from build123d import *
from OCP.BRepFilletAPI import BRepFilletAPI_MakeChamfer

# Parameters (mm, degrees)
BOSS_EXTRUDE1_DEPTH = 4.7625
CHAMFER1_SIZE       = 1.524
CHAMFER1_SIZE2      = 3.81
FILLET1_R           = 5.08


with BuildPart() as part:
    # Sketch1 → Boss-Extrude1 (new body)
    with BuildSketch(Plane.XY):
        with BuildLine():
            Line((-16.586093498, 9.370378993), (-35.326851484, -23.801808003))
            Line((-35.326851484, -23.801808003), (-2.154664488, -42.542565989))
            Line((-2.154664488, -42.542565989), (16.586093498, -9.370378993))
            ThreePointArc((16.586093498, -9.370378993), (9.370378993, 16.586093498), (-16.586093498, 9.370378993))
        make_face()
    extrude(amount=BOSS_EXTRUDE1_DEPTH)

    # Chamfer1: one chamfer whose edges measure the first distance from different faces: ONE call of the kernel's chamfer builder (chamfer() names one face for all edges)
    chamfer1_edges_1 = [part.edges().sort_by_distance(p)[0] for p in [
        (7.215714505, -25.956472491, 4.7625),
    ]]
    chamfer1_side_1 = [part.faces().sort_by_distance(p)[0] for p in [
        (7.215714505, -25.956472491, 2.38125),
    ]]
    chamfer1_edges_2 = [part.edges().sort_by_distance(p)[0] for p in [
        (9.370378993, 16.586093498, 4.7625),
    ]]
    chamfer1_side_2 = [part.faces().sort_by_distance(p)[0] for p in [
        (9.370378993, 16.586093498, 2.38125),
    ]]
    chamfer1_edges_3 = [part.edges().sort_by_distance(p)[0] for p in [
        (-25.956472491, -7.215714505, 4.7625),
    ]]
    chamfer1_side_3 = [part.faces().sort_by_distance(p)[0] for p in [
        (-25.956472491, -7.215714505, 2.38125),
    ]]
    chamfer1 = BRepFilletAPI_MakeChamfer(part.part.solid().wrapped)
    for e in chamfer1_edges_1:
        chamfer1.Add(CHAMFER1_SIZE, CHAMFER1_SIZE2, e.wrapped, chamfer1_side_1[0].wrapped)  # the first distance lies on this face
    for e in chamfer1_edges_2:
        chamfer1.Add(CHAMFER1_SIZE, CHAMFER1_SIZE2, e.wrapped, chamfer1_side_2[0].wrapped)  # the first distance lies on this face
    for e in chamfer1_edges_3:
        chamfer1.Add(CHAMFER1_SIZE, CHAMFER1_SIZE2, e.wrapped, chamfer1_side_3[0].wrapped)  # the first distance lies on this face
    add(Compound.cast(chamfer1.Shape()), mode=Mode.REPLACE)

    # Fillet1
    fillet1_edges = [part.edges().sort_by_distance(p)[0] for p in [
        (-35.326851484, -23.801808003, 1.61925),
        (-2.154664488, -42.542565989, 1.61925),
    ]]
    fillet(fillet1_edges, radius=FILLET1_R)


solid = part.part
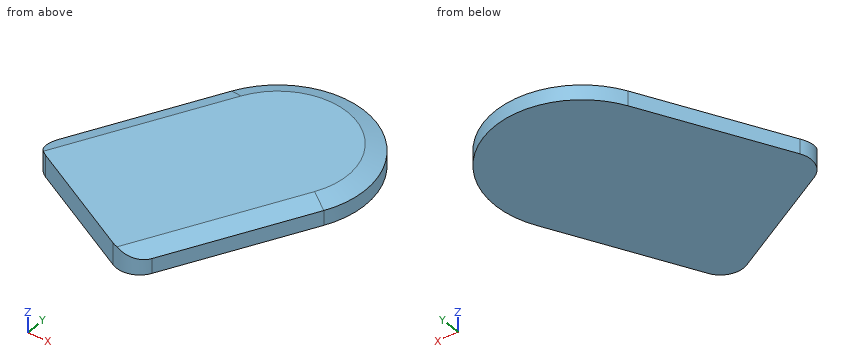
Source: CAD feature listing. Evaluate the final solid. Frame: model axes, mm. Coordinates: 2 decimals unless noted, no trailing zeros. Loops run counter-clockwise (first coordinate to the right, second up) from the corner with the lowest first, then second, coordinate; pieces in that order, holes last. Notation, with made-up numbers: (32, -11.5) - (62, -11.5) arc R21 ccw to (62, -0.5) - close; hole circle Ø1 at (40.25, -7). An arc over 180 degrees is marked (long way). One line per question, with ' | ' between items.
1) Section B-B, the plane y = 0. Return loops of the section in (x, z).
Report:
outline: (-21.88, 0) - (19.05, 0) - (19.05, 3.24) - (15.24, 4.76) - (-17.5, 4.76) - (-21.88, 3.24) - close
2) Line query: line 1 along Y through (x, z) = (-30, 2.95); line 2 along Y through (x, z) = (-27.5, 2.9); line 3 along X through (y, z) = (-35, 1.45). Output: solid intervals per line, ascending.
Report:
line 1: y = -26.81 to -14.37 | line 2: y = -28.22 to -9.95 | line 3: x = -15.51 to 2.11
3) First-contact query: P1, Ø2, axis at x = 1, z = 0.5, coming from the -Y side; P2, Ø1, axis at y = 13, z = 2, coming from the -X side; P3, Ø2, axis at x = 2, z = 3.5, coming from the +Y side. Flat tips, straight axial feed; report the tip coordinate or a pass-through.
Report:
P1: stops at y = -38.65 | P2: stops at x = -14.38 | P3: stops at y = 19.02
4) Section D-D, the plane y = -29.5. Return loops of the section in (x, z).
Report:
outline: (-25.24, 0) - (5.21, 0) - (5.21, 3.24) - (0.84, 4.76) - (-25.24, 4.76) - close
5) Section C-C, the plane x = -21. Return loops of the section in (y, z).
Report:
outline: (-31.9, 0) - (1.56, 0) - (1.56, 3.24) - (-6.19, 4.76) - (-31.9, 4.76) - close
6) Section A-A, the plane z = 2.5. Return loops of the section in (x, y), then the cut area to 3 significant figures.
Report:
outline: (-32.83, -19.38) arc R5.08 ccw to (-30.9, -26.3) - (-6.58, -40.04) arc R5.08 ccw to (0.34, -38.12) - (16.59, -9.37) arc R19.05 ccw to (-16.59, 9.37) - close | area: 2,010 mm²
